For this review, use the dimensioned drawing (mm, ordinates from the lowest corner) and the shaded views. A direction names the side the tool comes from. Coordinates: 2 decimals unless noted, no trailing zeros. Order: outer loops, then holes, each group sorted by start corner. A loop starts at its lowest first (then second) coordinate and runs counter-clockwise, first axis right, second up. Notation, with made-up numbers: M 53.25,-39 L 63.25,-39 A10 cw 63.25,-35 Z; hole C 2,-26 d9. An arc over 180 degrees is marked long. One line per item, written item: value.
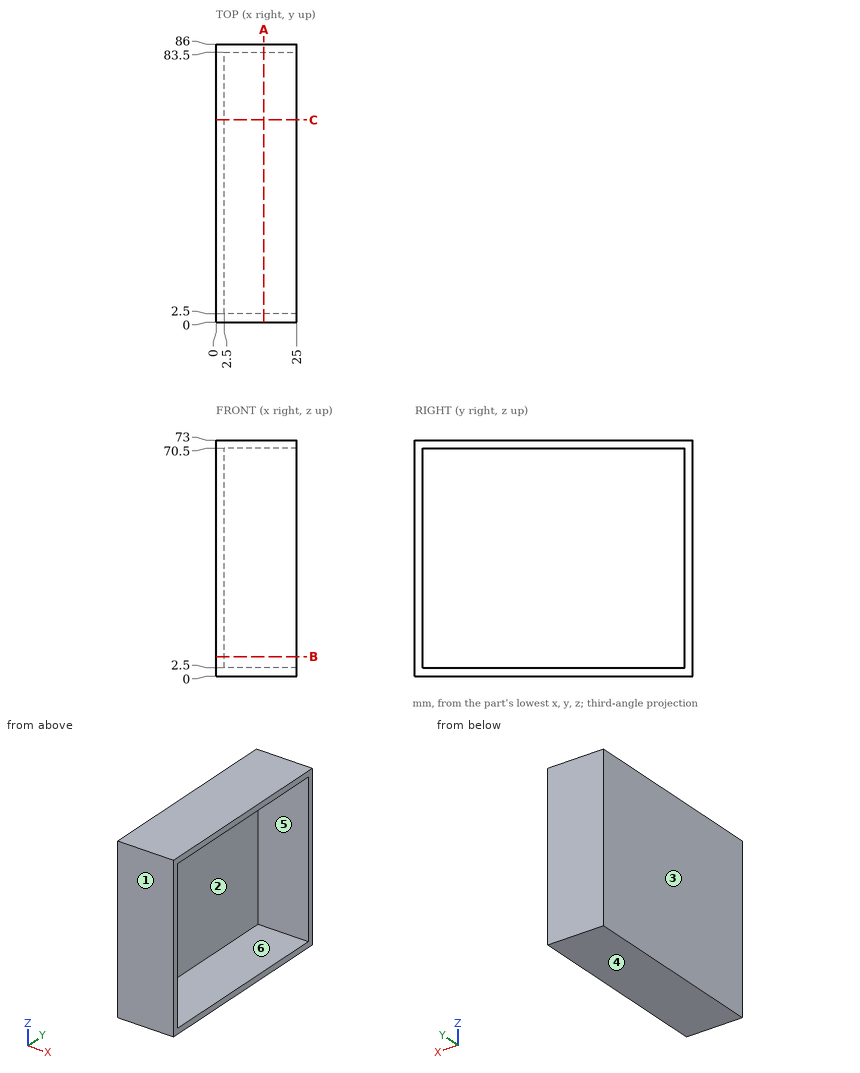
(1) We need section A-A, the plane x = 14.75. State the section outline as (y, z) points, plus the area to 3 significant figures.
Geometry results:
outline: M 0,0 L 86,0 L 86,73 L 0,73 Z; hole M 2.5,2.5 L 83.5,2.5 L 83.5,70.5 L 2.5,70.5 Z
area: 770 mm2
(2) We need section B-B, the plane z = 6. State the section outline as (x, y) points, plus the area to 4 significant figures.
Geometry results:
outline: M 0,0 L 25,0 L 25,2.5 L 2.5,2.5 L 2.5,83.5 L 25,83.5 L 25,86 L 0,86 Z
area: 327.5 mm2
(3) Tool access review of the marked faces 1 and 2: name each direction out of +Z, -Z, +X, -X, +Y, -Y from which nothing blocks a thin tool from reaching the whole face with its end or side.
Geometry results:
face 1: +Z, -Z, +X, -X, -Y
face 2: +X
(4) Mouldability with a two-part tool opening along Z and no side actions: class the marked faces 3, 4, 5 and 6 as +Z half, -Z half, draft (parallel to the pull), parting line (faces both ways), or undercut.
Geometry results:
face 3: draft
face 4: -Z half
face 5: undercut
face 6: undercut
(5) Insertion check: pin 1 Ø3 at (x, z) = (17.5, 57) entering from -Y; pin 2 Ø10 at (y, z) = (65.5, 33) entering from +X. Each pin has a flat end and moves straight along its axis. Give the tip position at first contact, or say it passes through.
Geometry results:
pin 1: stops at y = 0
pin 2: stops at x = 2.5
(6) For L1, parallel to Z at x = 12, y = 40; L2, parallel to Y at x = 7.5, z = 16.5; L3, parallel to X at y = 4, z = 68, list the stretches that pass through material, from the lowest coordinate up.
Geometry results:
L1: z = 0 to 2.5, 70.5 to 73
L2: y = 0 to 2.5, 83.5 to 86
L3: x = 0 to 2.5
(7) We need section C-C, the plane y = 62.5. State the section outline as (x, z) points, plus the area to 3 significant figures.
Geometry results:
outline: M 0,0 L 25,0 L 25,2.5 L 2.5,2.5 L 2.5,70.5 L 25,70.5 L 25,73 L 0,73 Z
area: 295 mm2
